```python
from build123d import *

# Parameters (mm, degrees)
F2_T     = -2.54
F3_R     = 58.705538
F4_DEPTH = 1.778


with BuildPart() as f1:
    # F0 (on Top) → F1 (revolve)
    with BuildSketch(Plane.XY):
        Polygon((66.235654, 49.231492), (0, 49.231492), (0, 40.974639), (85.226417, 40.974639), align=None)
    revolve(axis=Axis((0, 45.103066, 0), (0, 1, 0)))

    # F2
    f2_openings = [f1.faces().sort_by_distance(p)[0] for p in [
        (0, 40.974639, 0),
    ]]
    offset(amount=F2_T, openings=f2_openings)

    # F3 (on face) → F4 (join)
    with BuildSketch(Plane(origin=(0, 49.231492, 0), x_dir=(-1, 0, 0), z_dir=(0, 1, 0))):
        Circle(F3_R)
    extrude(amount=F4_DEPTH)


solid = f1.part
```
Geometry: final body of the model. Coordinates: model frame, mm. A direction names the side the tool comes from. Give positions to 0.01 mm unless a question says otherwise; leave off trailing zeros. Order: outer loops, then holes, each group sorted by start corner. A loop starts at its lowest first (then second) coordinate and runs counter-clockwise, first axis right, second up. Notation, with made-up numbers: (73, 21.5) -> (115, 21.5) arc R23 ccw to (115, 45.5) -> close; hole circle Ø9 at (15, 42). An arc over 180 degrees is marked (long way). Write each question's results on one line, items separated by ' | '. Start each with the question number.
1) Line query: line 1 (Y direction, x = -51.5, z = 31); line 2 (Y direction, x = 19, z = 63); line 3 (X direction, y = 43, z = -15). Output: solid intervals per line, ascending. Write a range as from..to.
2) First-contact query: pin 1 (1.5 mm diameter, centred on y = 45, z = -14.5, fed in from +X); pin 2 (12 mm diameter, centred on x = -47, z = 40, fed in from -Y); pin 3 (1.5 mm diameter, centred on x = -22.5, y = 45, fed in from -Z). Flat tips, straight axial feed; report the tip coordinate or a pass-through.
3) Draft query along X for faces 1 (the conical face through (-52.65, 46.414, 40.37)), 2 (the flat face through (-5, 49.231, 59)), 3 (the cylindrical face through (-27.09, 50.11, -52.08)). Return one class per face: pulls with the +X half, pulls with the -X half, needs draft (parallel to the pull), parting line crosses it, or undercut.
4) Set-up query: faces 4 (the flat face through (-1, 46.691, -1)), 5 (the conical face through (64.06, 48.83, -20.17)). Return all of +Z, -Z, +X, -X, +Y, -Y with unobstructed straight access to the full face (end or side cutting, diameter ignored); none if empty.
5) Section A-A (x = 0). Return loops of the section in (y, z), then the cut area to 3 significant figures.
6) Section B-B (z = 0). Return loops of the section in (x, y), then the cut area to 3 significant figures.
Calculated:
1) line 1: 46.69..49.23 | line 2: 46.65..49.23 | line 3: -79.16..-72.67, 72.67..79.16
2) pin 1: x = 76.33 | pin 2: y = 45.82 | pin 3: z = -74.38
3) face 1: undercut | face 2: needs draft | face 3: parting line crosses it
4) face 4: -Y | face 5: +Y
5) outline: (40.97, -85.23) -> (49.23, -66.24) -> (49.23, -58.71) -> (51.01, -58.71) -> (51.01, 58.71) -> (49.23, 58.71) -> (49.23, 66.24) -> (40.97, 85.23) -> (40.97, 78.86) -> (46.69, 65.71) -> (46.69, -65.71) -> (40.97, -78.86) -> close | area: 633 mm2
6) outline: (-85.23, 40.97) -> (-78.86, 40.97) -> (-65.71, 46.69) -> (65.71, 46.69) -> (78.86, 40.97) -> (85.23, 40.97) -> (66.24, 49.23) -> (58.71, 49.23) -> (58.71, 51.01) -> (-58.71, 51.01) -> (-58.71, 49.23) -> (-66.24, 49.23) -> close | area: 633 mm2
